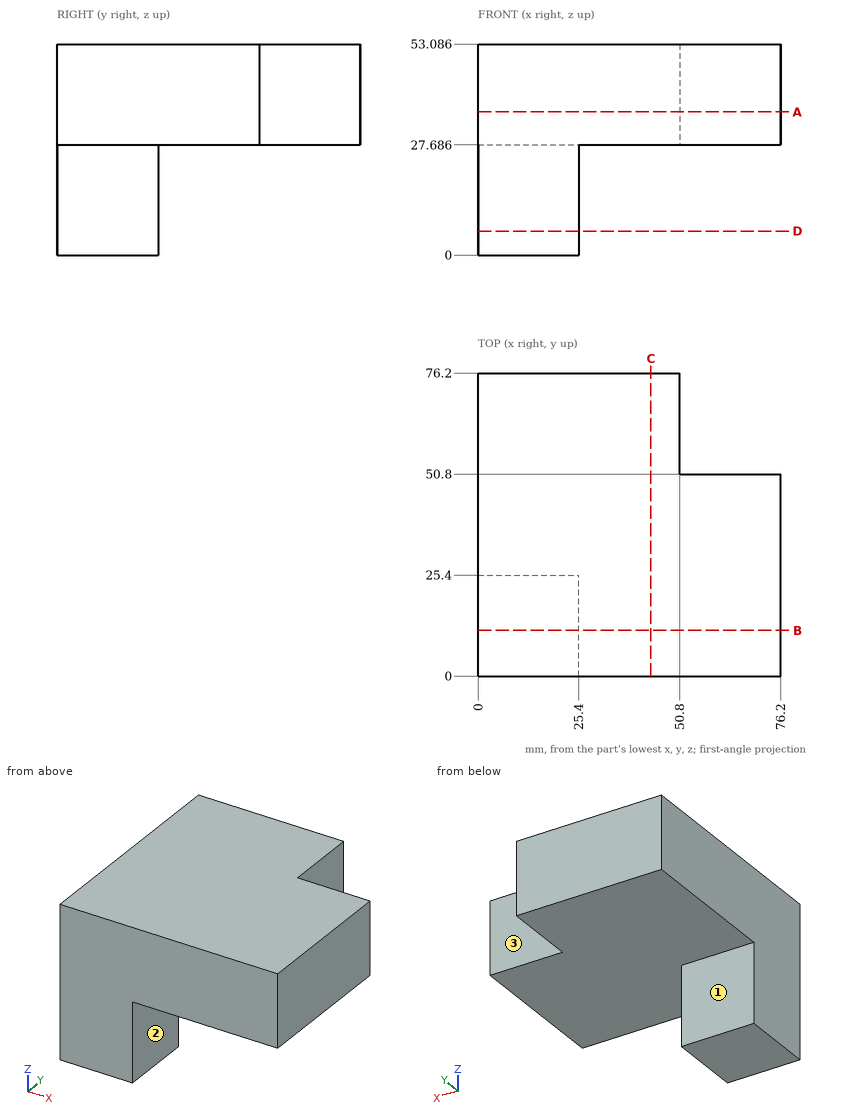
Answer from the drawing. Dimensions are ordinates in mm from the lowest x, y and z of the part. A direction names the side the tool comes from. Coordinates: 2 decimals unless noted, no trailing zeros. Write each loop counter-clockwise with the first axis right and the second up, starting at its lowest first coordinate (ties: lowest second). Pieces come first, ordered by that corner, then holes. Notation, with made-up numbers: (-3.5, 13) - (34.5, 13) arc R22 ccw to (34.5, 19) - close; hole circle Ø7 at (29, -23). An arc over 180 degrees is marked (long way). Return JSON: item names as keys, results as strings. Group by question number.
Q1. Find the intervals of material crossed by line 1 along Z through (x, y) = (27.5, 54.5); line 2 along Y through (x, z) = (18.5, 25.5), in increasing order. Write a range as [from, to].
Q2. Flat-ended cylindrical pins translate along their axes: pin 1 Ø20.5 at (y, z) = (66, 36) entering from +X; pin 2 Ø6 at (x, z) = (14.5, 10) entering from +Y. Find the tip coordinate at first contact, or state that the pin passes through.
Q3. The part is cut by section D-D on z = 6. Write down the section's boundary in (x, y), and give its area (3 significant figures).
Q4. The part is cut by section A-A on z = 36. Write down the section's boundary in (x, y), and give its area (3 significant figures).
Q5. The part is cut by section B-B on y = 11.5. Write down the section's boundary in (x, z).
Q6. The part is cut by section C-C on x = 43.5. Write down the section's boundary in (y, z), and give its area (3 significant figures).
Q7. Which of the six approach directions +Z, -Z, +X, -X, +Y, -Y give full straight-line access (tool end or side, diameter ignored) to the marked faces 1, 2 and 3?
Evaluation:
{
 "1": {"line 1": "z = [27.69, 53.09]", "line 2": "y = [0, 25.4]"},
 "2": {"pin 1": "stops at x = 50.8", "pin 2": "stops at y = 25.4"},
 "3": {"outline": "(0, 0) - (25.4, 0) - (25.4, 25.4) - (0, 25.4) - close", "area": "645 mm2"},
 "4": {"outline": "(0, 0) - (76.2, 0) - (76.2, 50.8) - (50.8, 50.8) - (50.8, 76.2) - (0, 76.2) - close", "area": "5,160 mm2"},
 "5": {"outline": "(0, 0) - (25.4, 0) - (25.4, 27.69) - (76.2, 27.69) - (76.2, 53.09) - (0, 53.09) - close"},
 "6": {"outline": "(0, 27.69) - (76.2, 27.69) - (76.2, 53.09) - (0, 53.09) - close", "area": "1,940 mm2"},
 "7": {"face 1": "-Z, +X, -X, +Y", "face 2": "-Z, +X, +Y, -Y", "face 3": "+Z, -Z, +X, +Y"}
}
